```python
from build123d import *

# Parameters (mm, degrees)
F3_DEPTH = 4
F4_R     = 2
F5_DEPTH = 4
F6_SIZE  = 0.5


# Not quite as in the source:
# - the program builds the solid bodies; features that only make, move or delete a surface that nothing else refers to are left out


with BuildPart() as f3:
    # F2 (on Top) → F3 (new body)
    with BuildSketch(Plane.XY):
        Polygon((5.6807082187, -1.0309643387), (3.7331954171, 4.4041554595), (-1.9475128016, 5.4351197982), (-5.6807082187, 1.0309643387), (-3.7331954171, -4.4041554595), (1.9475128016, -5.4351197982), align=None)
    extrude(amount=-F3_DEPTH)

    # F4 (on face) → F5 (cut)
    with BuildSketch(Plane(origin=(0, 0, -4), x_dir=(1, 0, 0), z_dir=(0, 0, -1))):
        Circle(F4_R)
    extrude(amount=-F5_DEPTH, mode=Mode.SUBTRACT)

    # F6
    f6_edges = [f3.edges().sort_by_distance(p)[0] for p in [
        (-0.892841, -4.919638, 0),
        (3.814111, -3.233042, 0),
        (4.706952, 1.686596, 0),
        (0.892841, 4.919638, 0),
        (-3.814111, 3.233042, 0),
        (-4.706952, -1.686596, 0),
    ]]
    chamfer(f6_edges, length=F6_SIZE)


solid = f3.part
```
CAD build for the part. Positions are in the model's coordinates, mm. Round coordinates to 2 decimals unless told otherwise and drop trailing zeros. Order: outer loops, then holes, each group sorted by start corner. A loop starts at its lowest first (then second) coordinate and runs counter-clockwise, first axis right, second up.
Q1. Slice it at B-B (x = 0.5). Write the cut outline in (y, z), and give its area (3 significant figures).
Q2. Slice it at C-C (y = 0). Write the cut outline in (x, z), and give its area (3 significant figures).
Q3. Slice it at A-A (z = -1.75). Write the cut outline in (x, y), and give its area (3 significant figures).
Q4. Two-plate mould, pull along Y, no slides. Class faces 1 (the cylindrical face through (0, 2, -2)), 2 (the flat face through (-3.79, 3.26, -2.23)), 3 (the flat face through (2.2, 0.1, 0)): pulls with the +Y half, pulls with the -Y half, needs draft (parallel to the pull), parting line crosses it, or undercut.
Q5. Slice it at D-D (x = 4.25). Write the cut outline in (y, z), and give its area (3 significant figures).
Q6. Wall check: L1, parallel to X at y = 0, z = -2.2; L2, parallel to X at y = -1.75, z = -2.15; L3, parallel to Y at x = 0, z = -2. Give the ranges that are in metal, low to high.
Results below:
1. outline: (-5.17, -4) - (-1.94, -4) - (-1.94, 0) - (-4.66, 0) - (-5.17, -0.5) - close; (1.94, -4) - (4.99, -4) - (4.99, -0.5) - (4.48, 0) - (1.94, 0) - close
1. area: 24.9 mm2
2. outline: (-5.31, -4) - (-2, -4) - (-2, 0) - (-4.78, 0) - (-5.31, -0.5) - close; (2, -4) - (5.31, -4) - (5.31, -0.5) - (4.78, 0) - (2, 0) - close
2. area: 26.2 mm2
3. outline: (-5.68, 1.03) - (-3.73, -4.4) - (1.95, -5.44) - (5.68, -1.03) - (3.73, 4.4) - (-1.95, 5.44) - close; hole circle Ø4 at (0, 0)
3. area: 74.0 mm2
4. face 1: undercut
4. face 2: pulls with the +Y half
4. face 3: needs draft
5. outline: (-2.72, -4) - (2.96, -4) - (2.96, -0.5) - (1.48, 0) - (-1.95, 0) - (-2.72, -0.5) - close
5. area: 22.2 mm2
6. L1: x = -5.31 to -2, 2 to 5.31
6. L2: x = -4.68 to -0.97, 0.97 to 5.07
6. L3: y = -5.08 to -2, 2 to 5.08
